The model under review builds one solid part; all positions refer to its coordinate system, in mm. Face numbers are marked on the shaded views. Round coordinates to 2 decimals unless told otherwise and drop trailing zeros. Order: outer loops, then holes, each group sorted by start corner. A loop starts at its lowest first (then second) coordinate and runs counter-clockwise, first axis right, second up. Notation, with made-up numbers: M -18.5,-16.5 L -8.5,-16.5 A23 ccw -8.5,4.5 Z; hole C 1,-2.5 d10. An arc over 180 degrees is marked long. Answer as a JSON object with one key per item and string values. Group by question number.
1. To check wall thickness, follow probe 1 along Z at (x, y) = (-6.5, 5.5); probe 2 along X at (y, z) = (7, -3); probe 3 along Z at (x, y) = (51.5, 6.75). State the ranges of each line that lie inside material, in increasing order. Write a range as [from, to].
2. Add section B-B on x = 44. State the section outline as (y, z) points.
3. Add section C-C on x = -3.5. State the section outline as (y, z) points, and give its area (3 significant figures).
4. Mouldability with a two-part tool opening along Z and no side actions: class the marked faces 1, 2, 3 and 4 as released by +Z, released by -Z, zero draft, split by the parting line, or undercut.
5. Add section D-D on z = 43.5. State the section outline as (x, y) points.
6. Add section A-A on y = 3.75. State the section outline as (x, z) points, and give its area (3 significant figures).
7. Clearance check with flat-ended pins moving along their axes: P1, Ø3, axis at y = 3, z = 5.5, coming from the +X side; P2, Ø5, axis at x = -7.5, y = 3, coming from the +Z side; P3, Ø2, axis at y = 4, z = -2.5, coming from the +X side. State where each tip first meets the part, or that it passes through.
```python
from build123d import *

# Parameters (mm, degrees)
BOSS_EXTRUDE1_DEPTH = 9
FILLET1_R           = 8
FILLET2_R           = 3


with BuildPart() as part:
    # Sketch1 → Boss-Extrude1 (new body)
    with BuildSketch(Plane(origin=(0, 0, 0), x_dir=(1, 0, 0), z_dir=(0, 1, 0))):
        Polygon((35, 0), (63.867513459, -50), (28.867513459, -50), (0, 0), align=None)
        Polygon((-65, 0), (0, 0), (35, 0), (55, 0), (55, 7), (-65, 7), align=None)
    extrude(amount=BOSS_EXTRUDE1_DEPTH)

    # Fillet1
    fillet1_edges = [part.edges().sort_by_distance(p)[0] for p in [
        (35, 4.5, 0),
    ]]
    fillet(fillet1_edges, radius=FILLET1_R)

    # Fillet2
    fillet2_edges = [part.edges().sort_by_distance(p)[0] for p in [
        (63.867513459, 4.5, 50),
        (28.867513459, 4.5, 50),
        (0, 4.5, 0),
    ]]
    fillet(fillet2_edges, radius=FILLET2_R)


solid = part.part
```
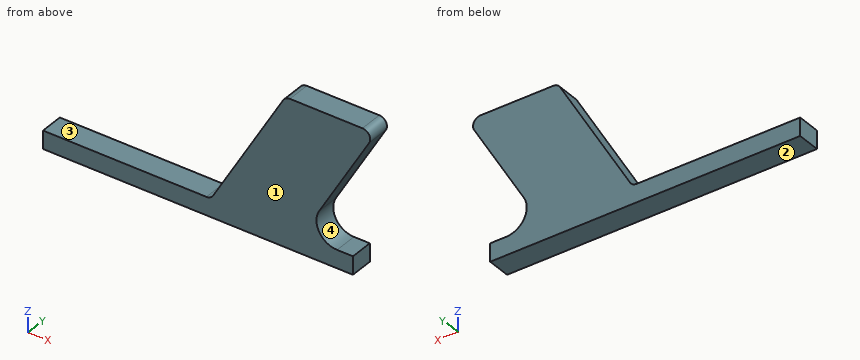
Recorded:
{
 "1": {"probe 1": "z = [-7, 0]", "probe 2": "x = [-65, 55]", "probe 3": "z = [-7, 0], [28.58, 50]"},
 "2": {"outline": "M 0,-7 L 9,-7 L 9,1.64 L 0,1.64 Z; M 0,15.59 L 9,15.59 L 9,50 L 0,50 Z"},
 "3": {"outline": "M 0,-7 L 9,-7 L 9,0 L 0,0 Z", "area": "63.0 mm²"},
 "4": {"face 1": "zero draft", "face 2": "released by -Z", "face 3": "released by +Z", "face 4": "undercut"},
 "5": {"outline": "M 25.11,0 L 60.11,0 L 60.11,9 L 25.11,9 Z"},
 "6": {"outline": "M -65,-7 L 55,-7 L 55,0 L 48.86,0 A8 cw 41.93,12 L 61.27,45.5 A3 ccw 58.67,50 L 30.6,50 A3 ccw 28,48.5 L 0.87,1.5 A3 cw -1.73,0 L -65,0 Z", "area": "2,630 mm²"},
 "7": {"P1": "stops at x = 41.93", "P2": "stops at z = 0", "P3": "stops at x = 55"}
}
